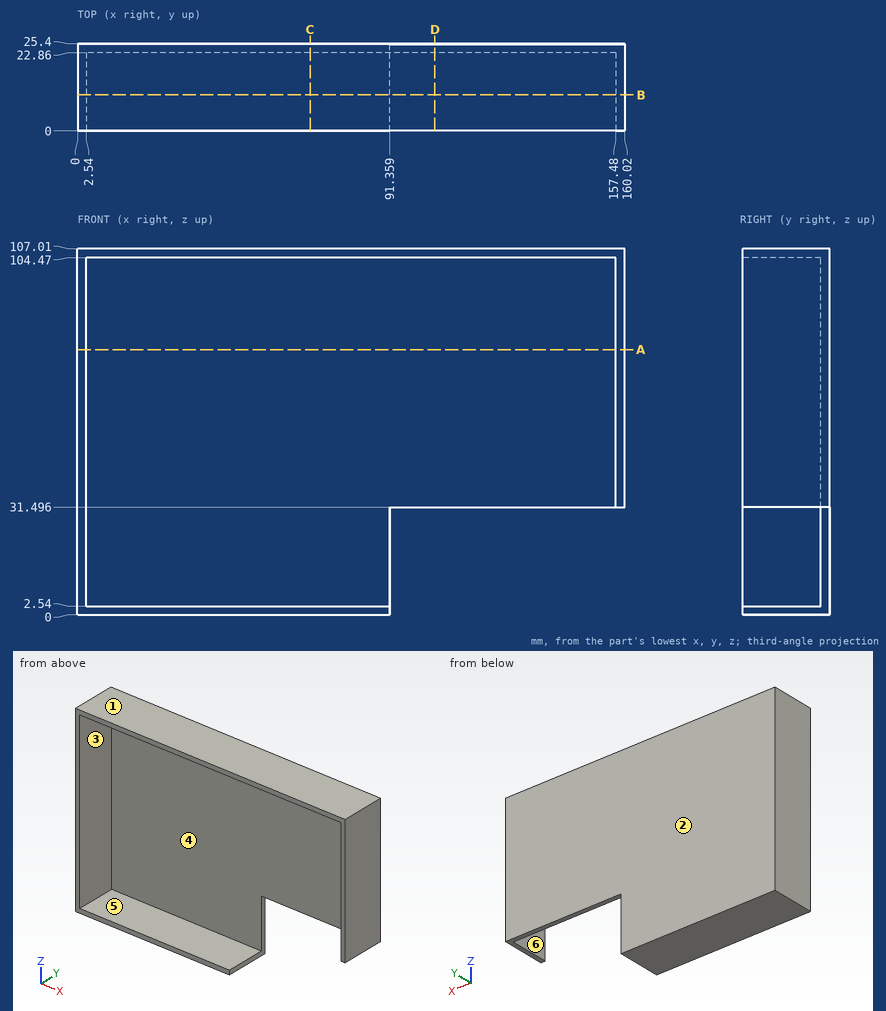
Here's the drawing with two shaded views (mm, measured from the low corner). I have some questions. A direction names the side the tool comes from. Give positions to 0.01 mm unless a question says otherwise; leave off trailing zeros. Write each loop counter-clockwise with the first axis right and the second up, starting at its lowest first coordinate (ties: lowest second). Pieces come first, ordered by that corner, then holes. Notation, with made-up numbers: (71.5, 89) -> (106.5, 89) arc R30 ccw to (106.5, 120) -> close; hole circle Ø10 at (11.5, 49.5). An arc over 180 degrees is marked (long way). Answer as a JSON object with one key per item and string values. Group by question number.
Item 1: Suppose I cut it at C-C (x = 68). Please give me the cut outline in (y, z), plus the area to 3 significant figures.
Item 2: Suppose I cut it at D-D (x = 104.5). Please give me the cut outline in (y, z), plus the area to 3 significant figures.
Item 3: We'd pull the mould along Z, two halves only. Please class the marked faces 1, 2 and 3: +Z half, -Z half, draft (parallel to the pull), parting line (faces both ways), or undercut.
Item 4: Suppose I cut it at B-B (y = 10.5). Please give me the cut outline in (x, z), plus the area to 3 significant figures.
Item 5: I'm going to push flat-ended pins straight in: P1, Ø7.5, axis at y = 14.5, z = 20.5, coming from the +X side; P2, Ø12.5, axis at x = 137.5, y = 17.5, coming from the -Z side. Where does each tip first touch, or does it pass through?
Item 6: Suppose I cut it at A-A (z = 77.5). Please give me the cut outline in (x, y).
Item 7: Please list where these lines run through material, in increasing order: line 1 (Z direction, x = 75, y = 1); line 2 (X direction, y = 7.5, z = 59); line 3 (Y direction, x = 36.5, z = 59). Write a range as [from, to].
Item 8: For the marked faces 4, 5 and 6, which set-ups out of +Z, -Z, +X, -X, +Y, -Y let a thin tool reach every point of the face, with its end or its side?
Findings:
{
 "1": {"outline": "(0, 0) -> (25.4, 0) -> (25.4, 107.01) -> (0, 107.01) -> (0, 104.47) -> (22.86, 104.47) -> (22.86, 2.54) -> (0, 2.54) -> close", "area": "388 mm²"},
 "2": {"outline": "(0, 104.47) -> (22.86, 104.47) -> (22.86, 31.5) -> (25.4, 31.5) -> (25.4, 107.01) -> (0, 107.01) -> close", "area": "250 mm²"},
 "3": {"face 1": "+Z half", "face 2": "draft", "face 3": "undercut"},
 "4": {"outline": "(0, 0) -> (91.36, 0) -> (91.36, 2.54) -> (2.54, 2.54) -> (2.54, 104.47) -> (157.48, 104.47) -> (157.48, 31.5) -> (160.02, 31.5) -> (160.02, 107.01) -> (0, 107.01) -> close", "area": "1,080 mm²"},
 "5": {"P1": "stops at x = 2.54", "P2": "stops at z = 31.5"},
 "6": {"outline": "(0, 0) -> (2.54, 0) -> (2.54, 22.86) -> (157.48, 22.86) -> (157.48, 0) -> (160.02, 0) -> (160.02, 25.4) -> (0, 25.4) -> close"},
 "7": {"line 1": "z = [0, 2.54], [104.47, 107.01]", "line 2": "x = [0, 2.54], [157.48, 160.02]", "line 3": "y = [22.86, 25.4]"},
 "8": {"face 4": "-Y", "face 5": "+X, -Y", "face 6": "-Z, -Y"}
}
